Check sheet for the modelled part. Datum: model origin and axes. Units: mm. Face numbers are marked on the shaded views. Give positions to 0.01 mm unless a question says otherwise; leave off trailing zeros. Loops run counter-clockwise (first coordinate to the right, second up) from the corner with the lowest first, then second, coordinate; pieces in that order, holes last. Notation, with made-up numbers: (79, 61) - (86, 61) arc R21 ccw to (86, 80) - close; hole circle Ø7 at (1, 53). An arc over 180 degrees is marked (long way). Answer in a Markdown table with one row per item. Add a question column.
(1) Sectioned sample at B-B on y = 6. Enter the section's corners in (x, z).
(2) Sectioned sample at C-C on z = -6.5. Enter the section's corners in (x, y).
(3) Sectioned sample at A-A on z = 5. Enter the section's corners in (x, y), then the cut area to 3 significant figures.
(4) Thickness scan on L1, parallel to X at y = -11.1, z = 5; L2, parallel to Z at x = 28.8, y = 1; L3, parallel to X at y = 13.5, z = -30. Record the ranges inside material, lowest first.
(5) Go/stop test with flat-tipped pins: P1, Ø1, axis at x = 41, y = -11, coming from the -Z side; P2, Ø1.8, axis at x = 39.5, z = 5.5, coming from the +Y side; P3, Ø0.6, axis at x = 29, z = -25, coming from the -Y side; P4, Ø10, axis at x = -19.5, z = 2.5, coming from the -Y side. Record where each tip stops, or that it passes through.
(6) Sectioned sample at D-D on z = -20. Enter the section's corners in (x, y), then the cut area to 3 significant figures.
(7) Draft check along X on the marked faces 1, 2 and 3. Enter one of: released by +X, released by -X, zero draft, split by the parting line, or undercut.
from build123d import *

# Parameters (mm, degrees)
EXTRUDE_1_DEPTH     = 1.5
EXTRUDE_2_DEPTH     = 1.5
SKETCH_3_W          = 6
SKETCH_3_H          = 2
EXTRUDE_3_DEPTH     = 6
SKETCH_4_R          = 1.55
CUT_EXTRUDE_1_DEPTH = 4.5
SKETCH_5_W          = 2
SKETCH_5_H          = 20
EXTRUDE_4_DEPTH     = 35
SKETCH_6_R          = 1.55
CUT_EXTRUDE_2_DEPTH = 35
SKETCH_7_R          = 2.55
CUT_EXTRUDE_4_DEPTH = 35


with BuildPart() as part:
    # 草图1 → 凸台-拉伸1 (new body)
    with BuildSketch(Plane.XY):
        Polygon((-30, 12), (-30, -12), (30, -12), (30, 12), (30, 16), (-30, 16), align=None)
    extrude(amount=EXTRUDE_1_DEPTH)

    # 草图2 → 凸台-拉伸2 (add)
    with BuildSketch(Plane.XY.offset(1.5)):
        Polygon((-40, -7), (-30, -7), (-27, -7), (-27, -12), (-30, -12), (-40, -12), align=None)
        Polygon((40, -7), (40, -12), (30, -12), (27, -12), (27, -7), (30, -7), align=None)
    extrude(amount=-EXTRUDE_2_DEPTH)

    # 草图3 → 凸台-拉伸3 (add)
    with BuildSketch(Plane.XY.offset(1.5)):
        with Locations((39, -11)):
            Rectangle(SKETCH_3_W, SKETCH_3_H)
        with Locations((-39, -11)):
            Rectangle(SKETCH_3_W, SKETCH_3_H)
    extrude(amount=EXTRUDE_3_DEPTH)

    # 草图4 → 切除-拉伸1 (cut)
    with BuildSketch(Plane.XZ.offset(12)):
        with Locations(Location((39, 5, 0), (0, 0, 270))):
            Circle(SKETCH_4_R)
        with Locations(Location((-39, 5, 0), (0, 0, 270))):
            Circle(SKETCH_4_R)
    extrude(amount=-CUT_EXTRUDE_1_DEPTH, mode=Mode.SUBTRACT)

    # 草图5 → 凸台-拉伸4 (add)
    with BuildSketch(Plane(origin=(0, 0, 0), x_dir=(-1, 0, 0), z_dir=(0, 0, -1))):
        with Locations((29, 6)):
            Rectangle(SKETCH_5_W, SKETCH_5_H)
        with Locations((-29, 6)):
            Rectangle(SKETCH_5_W, SKETCH_5_H)
    extrude(amount=EXTRUDE_4_DEPTH)

    # 草图6 → 切除-拉伸2 (cut)
    with BuildSketch(Plane(origin=(30, 0, 0), x_dir=(0, 0, -1), z_dir=(1, 0, 0))):
        with Locations((25, 6)):
            Circle(SKETCH_6_R)
        with Locations((30, 11)):
            Circle(SKETCH_6_R)
        with Locations(Location((30, 1, 0), (0, 0, 90))):
            Circle(SKETCH_6_R)
        with Locations(Location((20, 1, 0), (0, 0, 90))):
            Circle(SKETCH_6_R)
        with Locations((20, 11)):
            Circle(SKETCH_6_R)
    extrude(amount=-CUT_EXTRUDE_2_DEPTH, mode=Mode.SUBTRACT)

    # 草图7 → 切除-拉伸4 (cut)
    with BuildSketch(Plane.ZY.offset(30)):
        with Locations(Location((-25, 6, 0), (0, 0, 270))):
            Circle(SKETCH_7_R)
    extrude(amount=-CUT_EXTRUDE_4_DEPTH, mode=Mode.SUBTRACT)


solid = part.part
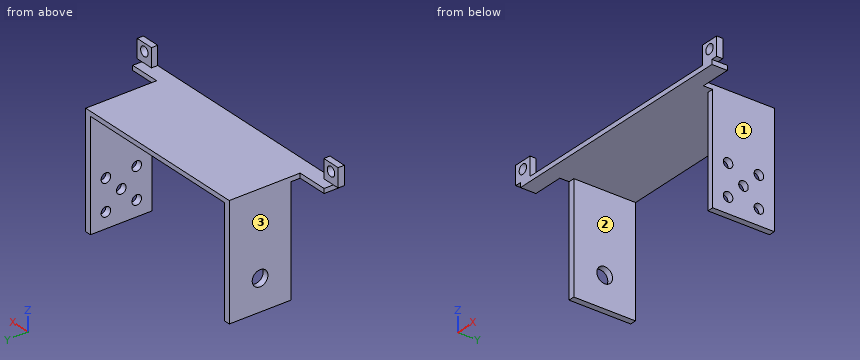
Reply:
| question | item | result |
|---|---|---|
| 1 | outline | (-30, -35) - (-28, -35) - (-28, -27.55) - (-30, -27.55) - close; (-30, -22.45) - (-28, -22.45) - (-28, 0) - (28, 0) - (28, -23.45) - (30, -23.45) - (30, 1.5) - (-30, 1.5) - close; (28, -35) - (30, -35) - (30, -26.55) - (28, -26.55) - close |
| 2 | outline | (-30, -4) - (-28, -4) - (-28, 16) - (-30, 16) - close; (28, -4) - (30, -4) - (30, 16) - (28, 16) - close |
| 3 | outline | (-42, -12) - (-40.55, -12) - (-40.55, -10) - (-42, -10) - close; (-37.45, -12) - (-36, -12) - (-36, -10) - (-37.45, -10) - close; (36, -12) - (37.45, -12) - (37.45, -10) - (36, -10) - close; (40.55, -12) - (42, -12) - (42, -10) - (40.55, -10) - close |
| 3 | area | 11.6 mm^2 |
| 4 | L1 | -42 to -40.55, -37.45 to -36, 36 to 37.45, 40.55 to 42 |
| 4 | L2 | -35 to -31.55, -28.45 to -21.55, -18.45 to 1.5 |
| 4 | L3 | -30 to -28, 28 to 30 |
| 5 | P1 | z = 1.5 |
| 5 | P2 | y = -10 |
| 5 | P3 | y = -4 |
| 5 | P4 | y = -12 |
| 6 | outline | (-30, -4) - (-28, -4) - (-28, 16) - (-30, 16) - close; (28, -4) - (30, -4) - (30, -0.55) - (28, -0.55) - close; (28, 2.55) - (30, 2.55) - (30, 9.45) - (28, 9.45) - close; (28, 12.55) - (30, 12.55) - (30, 16) - (28, 16) - close |
| 6 | area | 67.6 mm^2 |
| 7 | face 1 | released by +X |
| 7 | face 2 | undercut |
| 7 | face 3 | released by -X |
